Can you work these out from the model? Positions are in its coordinate system, mm. A direction names the side the tool comes from. Give positions to 0.01 mm unless a question says otherwise; leave off trailing zeros. Write each loop counter-clockwise with the first axis right and the second up, starting at its lowest first coordinate (ties: lowest second). Pieces come first, ordered by that corner, then holes.
1. If I drill on probe 1 along Y at (x, z) = (0, 1); probe 2 along X at (y, z) = (9.5, 3); probe 3 along X at (y, z) = (54, 5.5), over which ranges is the centre line in solid material (lowest first)?
2. Thinking about a two-plate mould opening in X: for faces 4 (the flat face through (2, 58, 6)), 5 (the cylindrical face through (-0.867, -57.905, 0.451)), 6 (the cylindrical face through (0, 64, 3)), which applies, pulls with the +X half, pulls with the -X half, needs draft (parallel to the pull), parting line crosses it, or undercut?
3. On a 3-axis mill with a long thin cutter (end or side, diameter ignored), from which of +Z, -Z, +X, -X, +Y, -Y can I reach the whole of each face in a straight line? I mean faces 1 (the flat face through (0, 54, 4)), 2 (the flat face through (-7, 22, 0)), 3 (the flat face through (-6, -1, 2)). Say none if no direction works.
4. Suppose I cut it at B-B (y = -32). Please give me the cut outline in (x, z).
5. Suppose I cut it at A-A (x = 0). Please give me the cut outline in (y, z), and give its area (3 significant figures).
6. I'm going to push flat-ended pins straight in: pin 1 (3 mm diameter, centred on x = 3, z = -1, fed in from +Y); pin 2 (6.5 mm diameter, centred on x = 0.5, y = 54, fed in from +Z); pin 3 (6 mm diameter, centred on x = 4.5, y = 15.5, fed in from -Z). Where does each tip first touch, or does it pass through?
7. Suppose I cut it at C-C (z = 2.5). Please give me the cut outline in (x, y).
```python
from build123d import *

# Parameters (mm, degrees)
CROQUIS1_R              = 4
SALIENTE_EXTRUIR1_DEPTH = 4
SALIENTE_EXTRUIR2_START = -3
CROQUIS1_5_R            = 4
SALIENTE_EXTRUIR2_DEPTH = 3
REDONDEO2_R             = 1
CROQUIS1_6_R            = 4
SALIENTE_EXTRUIR3_DEPTH = 6
REDONDEO1_R             = 10


with BuildPart() as part:
    # Croquis1 → Saliente-Extruir1 (new body)
    with BuildSketch(Plane.XY):
        with BuildLine():
            Line((10, 54), (10, -54))
            ThreePointArc((10, -54), (0, -64), (-10, -54))
            Line((-10, -54), (-10, 54))
            ThreePointArc((-10, 54), (0, 64), (10, 54))
        make_face()
        with Locations((0, -54)):
            Circle(CROQUIS1_R, mode=Mode.SUBTRACT)
        with BuildLine():
            Line((6, 38), (6, -38))
            ThreePointArc((6, -38), (0, -44), (-6, -38))
            Line((-6, -38), (-6, 38))
            ThreePointArc((-6, 38), (0, 44), (6, 38))
        make_face(mode=Mode.SUBTRACT)
    extrude(amount=SALIENTE_EXTRUIR1_DEPTH)

    # Croquis1<5> → Saliente-Extruir2 (add)
    with BuildSketch(Plane.XY.offset(SALIENTE_EXTRUIR2_START)):
        with BuildLine():
            Line((10, -54), (10, -47))
            Line((10, -47), (-10, -47))
            Line((-10, -47), (-10, -54))
            ThreePointArc((-10, -54), (0, -64), (10, -54))
        make_face()
        with Locations((0, -54)):
            Circle(CROQUIS1_5_R, mode=Mode.SUBTRACT)
    extrude(amount=SALIENTE_EXTRUIR2_DEPTH)

    # Redondeo2
    redondeo2_edges = [part.edges().sort_by_distance(p)[0] for p in [
        (0, -47, 0),
        (0, -47, -3),
    ]]
    fillet(redondeo2_edges, radius=REDONDEO2_R)

    # Croquis1<6> → Saliente-Extruir3 (add)
    with BuildSketch(Plane.XY):
        with BuildLine():
            Line((10, 47), (10, 54))
            ThreePointArc((10, 54), (0, 64), (-10, 54))
            Line((-10, 54), (-10, 47))
            Line((-10, 47), (10, 47))
        make_face()
        with Locations((0, 54)):
            Circle(CROQUIS1_6_R, mode=Mode.SUBTRACT)
    extrude(amount=SALIENTE_EXTRUIR3_DEPTH)

    # Redondeo1
    # the kernel refuses this fillet: 10 mm, written as the material it adds along each edge
    with BuildSketch(Plane(origin=(-10, 47, 4), x_dir=(0, 0, 1), z_dir=(1, 0, 0))) as redondeo1_piece_1_section:
        with BuildLine():
            CenterArc((10, 6), REDONDEO1_R, 180, 36.869897646)
            Line((0, 6), (-0.2, 6))
            Line((-0.2, 6), (-0.2, 0))
            Line((-0.2, 0), (0, -0.2))
            ThreePointArc((0, -0.2), (1, -0.2), (1.84, -0.12))
            Line((1.84, -0.12), (2, 0))
        make_face()
    redondeo1_piece_1 = extrude(amount=20, mode=Mode.PRIVATE)
    redondeo1_piece_1 = redondeo1_piece_1 - Plane(origin=(0, 38, 4.484524187), x_dir=(-1, 0, 0), z_dir=(0, 0, -1)) * Cylinder(6, 65, mode=Mode.PRIVATE)
    add(redondeo1_piece_1)


solid = part.part
```
Checks:
1. probe 1: y = -64 to -58, -50 to -44, 44 to 64
1. probe 2: x = -10 to -6, 6 to 10
1. probe 3: x = -10 to -4, 4 to 10
2. face 4: needs draft
2. face 5: undercut
2. face 6: parting line crosses it
3. face 1: +Z
3. face 2: -Z, +X, -X, +Y
3. face 3: +Z, -Z
4. outline: (-10, 0) - (-6, 0) - (-6, 4) - (-10, 4) - close; (6, 0) - (10, 0) - (10, 4) - (6, 4) - close
5. outline: (-64, -3) - (-58, -3) - (-58, 4) - (-64, 4) - close; (-50, -3) - (-48, -3) arc R1 ccw to (-47, -2) - (-47, -1) arc R1 cw to (-46, 0) - (-44, 0) - (-44, 4) - (-50, 4) - close; (44, 0) - (64, 0) - (64, 6) - (58, 6) - (58, 4) - (50, 4) - (50, 6) - (47, 6) arc R10 cw to (44, 4.46) - close
5. area: 176 mm2
6. pin 1: stops at y = 63.82
6. pin 2: stops at z = 4
6. pin 3: stops at z = 0
7. outline: (-10, -54) arc R10 ccw to (10, -54) - (10, 54) arc R10 ccw to (-10, 54) - close; hole (-6, -38) arc R6 ccw to (6, -38) - (6, 38) arc R6 ccw to (-6, 38) - close; hole circle Ø8 at (0, -54)
